from build123d import *

# Parameters (mm, degrees)
SCHIZZO1_W                    = 50
SCHIZZO1_H                    = 80
ESTRUSIONE_ESTRUSIONE1_DEPTH  = 4
SCHIZZO2_W                    = 4
SCHIZZO2_H                    = 2.857142857
SCHIZZO2_W_2                  = 7
ESTRUSIONE_ESTRUSIONE2_DEPTH  = 4
SCHIZZO3_W                    = 4
SCHIZZO3_H                    = 5.714285715
SCHIZZO3_W_2                  = 7
ESTRUSIONE_ESTRUSIONE3_DEPTH  = 4
RIPETIZIONE_A_L1_COUNT        = 6
RIPETIZIONE_A_L1_PITCH        = 11.428571
SCHIZZO4_W                    = 6.25
SCHIZZO4_H                    = 4
ESTRUSIONE_ESTRUSIONE4_DEPTH  = 4
RIPETIZIONE_A_L2_COUNT        = 4
RIPETIZIONE_A_L2_PITCH        = 12.5
SCHIZZO5_W                    = 61
SCHIZZO5_H                    = 88
ESTRUSIONE_ESTRUSIONE5_DEPTH  = 4
RACCORDO1_R                   = 10
TAGLIO_ESTRUSIONE1_DEPTH      = 112.323851892
TAGLIO_ESTRUSIONE1_DEPTH_BACK = 112.323851892
RACCORDO2_R                   = 10


with BuildPart() as part:
    # Schizzo1 → Estrusione-Estrusione1 (new body)
    with BuildSketch(Plane(origin=(0, 0, 0), x_dir=(0, 0, -1), z_dir=(1, 0, 0))):
        with Locations((25, 40)):
            Rectangle(SCHIZZO1_W, SCHIZZO1_H)
    extrude(amount=ESTRUSIONE_ESTRUSIONE1_DEPTH)

    # Schizzo2 → Estrusione-Estrusione2 (add)
    with BuildSketch(Plane(origin=(4, 0, 0), x_dir=(0, 0, -1), z_dir=(1, 0, 0))):
        with Locations((-2, 78.571428572)):
            Rectangle(SCHIZZO2_W, SCHIZZO2_H)
        with Locations((53.5, 78.571428572)):
            Rectangle(SCHIZZO2_W_2, SCHIZZO2_H)
        with Locations((53.5, 1.428571429)):
            Rectangle(SCHIZZO2_W_2, SCHIZZO2_H)
        with Locations((-2, 1.428571429)):
            Rectangle(SCHIZZO2_W, SCHIZZO2_H)
    extrude(amount=-ESTRUSIONE_ESTRUSIONE2_DEPTH)

    # Schizzo3 → Estrusione-Estrusione3 (add)
    with BuildSketch(Plane(origin=(4, 0, 0), x_dir=(0, 0, -1), z_dir=(1, 0, 0))):
        with Locations((-2, 68.571428572)):
            Rectangle(SCHIZZO3_W, SCHIZZO3_H)
        with Locations((53.5, 68.571428572)):
            Rectangle(SCHIZZO3_W_2, SCHIZZO3_H)
    estrusione_estrusione3 = extrude(amount=-ESTRUSIONE_ESTRUSIONE3_DEPTH)

    # Ripetizione a L1: Estrusione-Estrusione3 ×6
    with Locations(*[(0, -i * RIPETIZIONE_A_L1_PITCH, 0) for i in range(1, RIPETIZIONE_A_L1_COUNT)]):
        add(estrusione_estrusione3)

    # Schizzo4 → Estrusione-Estrusione4 (add)
    with BuildSketch(Plane(origin=(4, 0, 0), x_dir=(0, 0, -1), z_dir=(1, 0, 0))):
        with Locations((6.25, 82)):
            Rectangle(SCHIZZO4_W, SCHIZZO4_H)
        with Locations((6.25, -2)):
            Rectangle(SCHIZZO4_W, SCHIZZO4_H)
    estrusione_estrusione4 = extrude(amount=-ESTRUSIONE_ESTRUSIONE4_DEPTH)

    # Ripetizione a L2: Estrusione-Estrusione4 ×4
    with Locations(*[(0, 0, -i * RIPETIZIONE_A_L2_PITCH) for i in range(1, RIPETIZIONE_A_L2_COUNT)]):
        add(estrusione_estrusione4)

    # Schizzo5 → Estrusione-Estrusione5 (add)
    with BuildSketch(Plane(origin=(4, 0, 0), x_dir=(0, 0, -1), z_dir=(1, 0, 0))):
        Polygon((64, -11), (46.160080614, -44.552008529), (-54.590569466, 9.018062365), (-11, 91), (64, 91), align=None)
        with Locations((26.5, 40)):
            Rectangle(SCHIZZO5_W, SCHIZZO5_H, mode=Mode.SUBTRACT)
    extrude(amount=-ESTRUSIONE_ESTRUSIONE5_DEPTH)

    # Raccordo1
    raccordo1_edges = [part.edges().sort_by_distance(p)[0] for p in [
        (2, -44.552008529, -46.160080614),
        (2, 9.018062365, 54.590569466),
    ]]
    fillet(raccordo1_edges, radius=RACCORDO1_R)

    # Schizzo6 → Taglio-Estrusione1 (cut, two sides: drawn at the far end of the back side and taken through both)
    with BuildSketch(Plane(origin=(4, 0, 0), x_dir=(0, 0, -1), z_dir=(1, 0, 0)).offset(-TAGLIO_ESTRUSIONE1_DEPTH_BACK)):
        with BuildLine():
            Line((21.2, 26), (21.2, 15))
            ThreePointArc((21.2, 15), (21.639339828, 13.939339828), (22.7, 13.5))
            Line((22.7, 13.5), (27.7, 13.5))
            ThreePointArc((27.7, 13.5), (28.760660172, 13.939339828), (29.2, 15))
            Line((29.2, 15), (29.2, 26))
            ThreePointArc((29.2, 26), (28.760660172, 27.060660172), (27.7, 27.5))
            Line((27.7, 27.5), (22.7, 27.5))
            ThreePointArc((22.7, 27.5), (21.639339828, 27.060660172), (21.2, 26))
        make_face()
    extrude(amount=TAGLIO_ESTRUSIONE1_DEPTH + TAGLIO_ESTRUSIONE1_DEPTH_BACK, mode=Mode.SUBTRACT)

    # Raccordo2
    raccordo2_edges = [part.edges().sort_by_distance(p)[0] for p in [
        (2, 91, -64),
        (2, -11, -64),
        (2, 91, 11),
    ]]
    fillet(raccordo2_edges, radius=RACCORDO2_R)


solid = part.part
Geometry check sheet. Reference: the model listing, model coordinates, mm. Round coordinates to 2 decimals unless told otherwise and drop trailing zeros. Loops run counter-clockwise (first coordinate to the right, second up) from the corner with the lowest first, then second, coordinate; pieces in that order, holes last.
Item 1: Mould release check, pull along Y, two halves, no side actions. Record for faces 1 (the flat face through (2, 65.714, 2)), 2 (the cylindrical face through (1.97, 89.61, 10.08)): pulls with the +Y half, pulls with the -Y half, needs draft (parallel to the pull), parting line crosses it, or undercut.
Item 2: Cross-section at A-A on y = 51. Record the boundary of the cut face in (x, z), then the cut area to 3 significant figures.
Item 3: Thickness scan on line 1 (Z direction, x = 3.1, y = 81) (3 decimals); line 2 (Y direction, x = 1, z = -1); line 3 (Y direction, x = 1.3, z = -1.5). Record the ranges inside material, lowest first.
Item 4: Cross-section at D-D on z = 39. Record the boundary of the cut face in (x, y), then the cut area to 3 significant figures.
Item 5: Cross-section at C-C on y = -18. Record the boundary of the cut face in (x, z), then the cut area to 3 significant figures.
Item 6: Gauge pin test, flat ends, axial feed: pin 1 (1.2 mm diameter, centred on x = 1.5, y = -2, fed in from +Z); pin 2 (1.2 mm diameter, centred on x = 2, y = -3, fed in from +Z); pin 3 (1.2 mm diameter, centred on x = 1.5, z = -52, fed in from -Y); pin 4 (5 mm diameter, centred on y = 18, z = 12, fed in from -X). Record the tip position at first contact, or that the pin passes through.
Item 7: Cross-section at B-B on x = 3.2. Count the separate pieces of the cut face and the enclosed holes in it, then the cut area to 3 significant figures.
Answer sheet:
1. face 1: undercut
1. face 2: pulls with the +Y half
2. outline: (0, -64) - (4, -64) - (4, -57) - (0, -57) - close; (0, -50) - (4, -50) - (4, 0) - (0, 0) - close; (0, 4) - (4, 4) - (4, 32.27) - (0, 32.27) - close
2. area: 341 mm2
3. line 1: z = -64 to -57, -46.875 to -40.625, -34.375 to -28.125, -21.875 to -15.625, -9.375 to -3.125, 4 to 16.317
3. line 2: y = -20.54 to -4, 0 to 80, 84 to 91
3. line 3: y = -20.81 to -4, 0 to 80, 84 to 91
4. outline: (0, 0.73) - (4, 0.73) - (4, 38.34) - (0, 38.34) - close
4. area: 150 mm2
5. outline: (0, -60.28) - (4, -60.28) - (4, 3.78) - (0, 3.78) - close
5. area: 256 mm2
6. pin 1: stops at z = 35
6. pin 2: stops at z = 33.12
6. pin 3: stops at y = -34.7
6. pin 4: stops at x = 0
7. separate pieces: 1
7. enclosed holes: 25
7. area: 10,400 mm2
